The listing builds one solid part. Answer for the finished solid, in the listing's coordinates (mm). A direction names the side the tool comes from. Coordinates: 2 decimals unless noted, no trailing zeros. Order: outer loops, then holes, each group sorted by start corner. A loop starts at its lowest first (then second) coordinate and runs counter-clockwise, first axis right, second up.
```python
from build123d import *

# Parameters (mm, degrees)
BOSS_EXTRUDE1_DEPTH         = 4.7625
F_3_4_0_75_DIAMETER_HOLE1_D = 19.05
F_6_CLEARANCE_HOLE1_D       = 4.3053


with BuildPart() as part:
    # Sketch1 → Boss-Extrude1 (new body)
    with BuildSketch(Plane.XY.offset(-4.2926)):
        with BuildLine():
            Line((11.2395, 14.2875), (11.2395, 1.55575))
            ThreePointArc((11.2395, 1.55575), (11.462684633, 1.016934633), (12.0015, 0.79375))
            Line((12.0015, 0.79375), (134.0485, 0.79375))
            ThreePointArc((134.0485, 0.79375), (134.587315367, 1.016934633), (134.8105, 1.55575))
            Line((134.8105, 1.55575), (134.8105, 14.2875))
            ThreePointArc((134.8105, 14.2875), (136.670371939, 18.777628061), (141.1605, 20.6375))
            Line((141.1605, 20.6375), (144.494250007, 20.6375))
            ThreePointArc((144.494250007, 20.6375), (145.033065373, 20.860684631), (145.256250007, 21.399499996))
            Line((145.256250007, 21.399499996), (145.256250453, 83.375499964))
            ThreePointArc((145.256250453, 83.375499964), (145.033065866, 83.914315228), (144.494250605, 84.137499968))
            Line((144.494250605, 84.137499968), (141.16049997, 84.137499992))
            ThreePointArc((141.16049997, 84.137499992), (134.8105, 90.487500015), (141.1605, 96.8375))
            Line((141.1605, 96.8375), (144.49425, 96.8375))
            ThreePointArc((144.49425, 96.8375), (145.033065367, 97.060684633), (145.25625, 97.5995))
            Line((145.25625, 97.5995), (145.25625, 159.5755))
            ThreePointArc((145.25625, 159.5755), (145.033065367, 160.114315367), (144.49425, 160.3375))
            Line((144.49425, 160.3375), (141.1605, 160.3375))
            ThreePointArc((141.1605, 160.3375), (136.670371939, 162.197371939), (134.8105, 166.6875))
            Line((134.8105, 166.6875), (134.8105, 179.41925))
            ThreePointArc((134.8105, 179.41925), (134.587315367, 179.958065367), (134.0485, 180.18125))
            Line((134.0485, 180.18125), (12.0015, 180.18125))
            ThreePointArc((12.0015, 180.18125), (11.462684633, 179.958065367), (11.2395, 179.41925))
            Line((11.2395, 179.41925), (11.2395, 166.6875))
            ThreePointArc((11.2395, 166.6875), (9.379628061, 162.197371939), (4.8895, 160.3375))
            Line((4.8895, 160.3375), (1.55575, 160.3375))
            ThreePointArc((1.55575, 160.3375), (1.016934633, 160.114315367), (0.79375, 159.5755))
            Line((0.79375, 159.5755), (0.79375, 97.5995))
            ThreePointArc((0.79375, 97.5995), (1.016934633, 97.060684633), (1.55575, 96.8375))
            Line((1.55575, 96.8375), (4.8895, 96.8375))
            ThreePointArc((4.8895, 96.8375), (11.2395, 90.487500015), (4.88950003, 84.1375))
            Line((4.88950003, 84.1375), (1.555749996, 84.137499976))
            ThreePointArc((1.555749996, 84.137499976), (1.016934626, 83.91431534), (0.79375, 83.375499968))
            Line((0.79375, 83.375499968), (0.79375, 21.3995))
            ThreePointArc((0.79375, 21.3995), (1.016934633, 20.860684633), (1.55575, 20.6375))
            Line((1.55575, 20.6375), (4.8895, 20.6375))
            ThreePointArc((4.8895, 20.6375), (9.379628061, 18.777628061), (11.2395, 14.2875))
        make_face()
    extrude(amount=BOSS_EXTRUDE1_DEPTH)

    # 3/4 (0.75) Diameter Hole1 (through all)
    with Locations(Plane.XY.offset(0.4699)):
        with Locations((33.782, 19.685), (76.454, 31.496), (119.888, 19.685), (119.888, 52.07), (33.782, 52.07), (75.184, 84.455), (119.888, 84.455), (25.4, 122.2248), (57.15, 122.2248), (88.9, 122.2248), (120.65, 122.2248), (25.4, 160.3248), (57.15, 160.3248), (88.9, 160.3248), (120.65, 160.3248)):
            Hole(F_3_4_0_75_DIAMETER_HOLE1_D / 2)

    # #6 Clearance Hole1 (through all)
    with Locations(Plane.XY.offset(0.4699)):
        with Locations((25.4, 142.875), (73.025, 142.875), (127, 142.875), (73.025, 61.647038728), (25.4, 34.925), (127, 34.925)):
            Hole(F_6_CLEARANCE_HOLE1_D / 2)


solid = part.part
```
(1) Find section A-A (x = 57.15). Write down the section's boundary in (y, z).
(2) Each of these flat-tipped pins is pushed along its axis until it touches: pin 1 Ø1 at (x, z) = (3.5, -1.5) entering from -Y; pin 2 Ø11.5 at (x, y) = (119.888, 19.685) entering from -Z; pin 3 Ø1 at (y, z) = (88, -2.5) entering from -X; pin 4 Ø1.7 at (x, z) = (142.5, -3) entering from +Y. Where does it stop, or does it pass through?
(3) The mould has two halves that part along Y. Classify faces 4 (the face through (9.33, 18.827, -1.945)), 5 (the face through (145.256, 52, -2)), 6 (the face through (90.14, 131.67, -1.94)): released by +Y, released by -Y, zero draft, split by the parting line, or undercut.
(4) Find section B-B (y = 52.07). Write down the section's boundary in (x, z).
(5) Consider line 1 (Y direction, x = 88.9, z = -1.35); line 2 (Y direction, x = 120.65, z = -1.2); line 3 (Y direction, x = 119.5, z = -1.95). Determine where each line is inside the solid, lowest interval first.
(6) Find section D-D (z = -3). Give the number of separate pieces and of enclosed holes in the cut face, and give its area (3 significant figures).
(7) For faces 1 (the face through (110.803, 22.546, -1.945)), 2 (the face through (134.81, 8, -2)), 3 (the face through (11.24, 8, -2)), determine the directions among +Z, -Z, +X, -X, +Y, -Y from which every point of the face is accessible in a straight line to the end or side of a thin tool.
(8) Find section C-C (x = 120.65). Write down the section's boundary in (y, z).
Findings below:
1. outline: (0.79, -4.29) - (112.7, -4.29) - (112.7, 0.47) - (0.79, 0.47) - close; (131.75, -4.29) - (150.8, -4.29) - (150.8, 0.47) - (131.75, 0.47) - close; (169.85, -4.29) - (180.18, -4.29) - (180.18, 0.47) - (169.85, 0.47) - close
2. pin 1: stops at y = 20.64
2. pin 2: passes through
2. pin 3: stops at x = 10.49
2. pin 4: stops at y = 160.34
3. face 4: released by -Y
3. face 5: zero draft
3. face 6: undercut
4. outline: (0.79, -4.29) - (24.26, -4.29) - (24.26, 0.47) - (0.79, 0.47) - close; (43.31, -4.29) - (110.36, -4.29) - (110.36, 0.47) - (43.31, 0.47) - close; (129.41, -4.29) - (145.26, -4.29) - (145.26, 0.47) - (129.41, 0.47) - close
5. line 1: y = 0.79 to 112.7, 131.75 to 150.8, 169.85 to 180.18
5. line 2: y = 0.79 to 10.19, 29.18 to 42.58, 61.56 to 74.96, 93.95 to 112.7, 131.75 to 150.8, 169.85 to 180.18
5. line 3: y = 0.79 to 10.17, 29.2 to 42.55, 61.59 to 74.94, 93.97 to 112.77, 131.68 to 150.87, 169.78 to 180.18
6. separate pieces: 1
6. enclosed holes: 21
6. area: 20,500 mm2
7. face 1: +Z, -Z
7. face 2: +Z, -Z, +X, -Y
7. face 3: +Z, -Z, -X, -Y
8. outline: (0.79, -4.29) - (10.19, -4.29) - (10.19, 0.47) - (0.79, 0.47) - close; (29.18, -4.29) - (42.58, -4.29) - (42.58, 0.47) - (29.18, 0.47) - close; (61.56, -4.29) - (74.96, -4.29) - (74.96, 0.47) - (61.56, 0.47) - close; (93.95, -4.29) - (112.7, -4.29) - (112.7, 0.47) - (93.95, 0.47) - close; (131.75, -4.29) - (150.8, -4.29) - (150.8, 0.47) - (131.75, 0.47) - close; (169.85, -4.29) - (180.18, -4.29) - (180.18, 0.47) - (169.85, 0.47) - close
